Build history of the part. All positions in model axes, mm. Round coordinates to 2 decimals unless told otherwise and drop trailing zeros. Use a Markdown table: item, result. Add a question column.
Item 1: Probe L1, parallel to Z at x = -24.5, y = 2; L2, parallel to X at y = 2.5, z = -13.25; L3, parallel to Z at x = 23.5, y = 1.25. List the from-to ranges inside material, lowest first.
Item 2: Two-plate mould, pull along X, no slides. Class faces 1 (the face through (127, 5, 1)), 2 (the face through (-127, 5, 1)), 3 (the face through (-99.543, 4.829, -1.041)): released by +X, released by -X, zero draft, split by the parting line, or undercut.
Item 3: Slice it at A-A, the plane y = 3.75. State how many separate pieces and enclosed holes the cut face has, plus the area to 3 significant figures.
from build123d import *

# Parameters (mm, degrees)
SKETCH1_W                      = 254
SKETCH1_H                      = 114.3
BOSS_EXTRUDE1_DEPTH            = 9.525
F_3_8_CLEARANCE_HOLE1_D        = 9.8044
F_3_8_CLEARANCE_HOLE1_DEPTH    = 10
F_3_8_CLEARANCE_HOLE1_TIP      = 2.945538927
M2_5_CLEARANCE_HOLE3_D         = 3.1
M2_5_CLEARANCE_HOLE3_DEPTH     = 10
M2_5_CLEARANCE_HOLE3_TIP       = 0.931333959
FILLET1_R                      = 2
M3_CLEARANCE_HOLE4_D           = 3.4
M3_CLEARANCE_HOLE4_DEPTH       = 10
M3_CLEARANCE_HOLE4_TIP         = 1.021463052
SKETCH22_R                     = 8
CUT_EXTRUDE1_DEPTH             = 140.5917194
M3_CLEARANCE_HOLE5_D           = 3.6
M3_CLEARANCE_HOLE5_DEPTH       = 10
M3_CLEARANCE_HOLE5_TIP         = 1.081549114
M2_5_CLEARANCE_HOLE4_OUTLINE_R = 1.55
M2_5_CLEARANCE_HOLE4_DEPTH     = 9.525


# Read off the part's stored shape, not the designer's step: M2.5 Clearance Hole4
with BuildPart() as part:
    # Sketch1 → Boss-Extrude1 (new body)
    with BuildSketch(Plane(origin=(0, 0, 0), x_dir=(1, 0, 0), z_dir=(0, 1, 0))):
        Rectangle(SKETCH1_W, SKETCH1_H)
    extrude(amount=BOSS_EXTRUDE1_DEPTH)

    # 3/8 Clearance Hole1
    with Locations(Plane(origin=(0, 9.525, 0), x_dir=(1, 0, 0), z_dir=(0, 1, 0))):
        with Locations((112.7125, 42.8625), (112.7125, -42.8675), (-112.7175, 42.8625), (-112.7175, -42.8675)):
            Hole(F_3_8_CLEARANCE_HOLE1_D / 2, depth=F_3_8_CLEARANCE_HOLE1_DEPTH)
            with Locations((0, 0, -(F_3_8_CLEARANCE_HOLE1_DEPTH + F_3_8_CLEARANCE_HOLE1_TIP / 2))):  # 118° drill point
                Cone(0, F_3_8_CLEARANCE_HOLE1_D / 2, F_3_8_CLEARANCE_HOLE1_TIP, mode=Mode.SUBTRACT)

    # M2.5 Clearance Hole3
    with Locations(Plane(origin=(0, 9.525, 0), x_dir=(1, 0, 0), z_dir=(0, 1, 0))):
        with Locations((24.5, 19), (-24.5, -39), (24.5, -39), (-24.5, 19)):
            Hole(M2_5_CLEARANCE_HOLE3_D / 2, depth=M2_5_CLEARANCE_HOLE3_DEPTH)
            with Locations((0, 0, -(M2_5_CLEARANCE_HOLE3_DEPTH + M2_5_CLEARANCE_HOLE3_TIP / 2))):  # 118° drill point
                Cone(0, M2_5_CLEARANCE_HOLE3_D / 2, M2_5_CLEARANCE_HOLE3_TIP, mode=Mode.SUBTRACT)

    # Fillet1
    fillet1_edges = [part.edges().sort_by_distance(p)[0] for p in [
        (127, 4.7625, 57.15),
        (-127, 4.7625, 57.15),
        (-127, 4.7625, -57.15),
        (127, 4.7625, -57.15),
    ]]
    fillet(fillet1_edges, radius=FILLET1_R)

    # M3 Clearance Hole4
    with Locations(Plane(origin=(0, 9.525, 0), x_dir=(1, 0, 0), z_dir=(0, 1, 0))):
        with Locations((-90.2, -20.8), (-88.35, 29.15), (-58.8, 13.25), (-46, -20.8)):
            Hole(M3_CLEARANCE_HOLE4_D / 2, depth=M3_CLEARANCE_HOLE4_DEPTH)
            with Locations((0, 0, -(M3_CLEARANCE_HOLE4_DEPTH + M3_CLEARANCE_HOLE4_TIP / 2))):  # 118° drill point
                Cone(0, M3_CLEARANCE_HOLE4_D / 2, M3_CLEARANCE_HOLE4_TIP, mode=Mode.SUBTRACT)

    # Sketch22 → Cut-Extrude1 (cut, through all)
    with BuildSketch(Plane(origin=(0, 9.525, 0), x_dir=(1, 0, 0), z_dir=(0, 1, 0))):
        with Locations(Location((-107.475, 0, 0), (0, 0, 270))):
            Circle(SKETCH22_R)
    extrude(amount=-CUT_EXTRUDE1_DEPTH, mode=Mode.SUBTRACT)

    # M3 Clearance Hole5
    with Locations(Plane(origin=(0, 9.525, 0), x_dir=(1, 0, 0), z_dir=(0, 1, 0))):
        with Locations((61.84, 40.64), (61.84, -40.64), (82.16, -40.64), (82.16, 40.64)):
            Hole(M3_CLEARANCE_HOLE5_D / 2, depth=M3_CLEARANCE_HOLE5_DEPTH)
            with Locations((0, 0, -(M3_CLEARANCE_HOLE5_DEPTH + M3_CLEARANCE_HOLE5_TIP / 2))):  # 118° drill point
                Cone(0, M3_CLEARANCE_HOLE5_D / 2, M3_CLEARANCE_HOLE5_TIP, mode=Mode.SUBTRACT)

    # M2.5 Clearance Hole4 outline → M2.5 Clearance Hole4 (cut)
    with BuildSketch(Plane(origin=(0, 0, 0), x_dir=(1, 0, 0), z_dir=(0, 1, 0))):
        with Locations((-10.16, 6.35)):
            Circle(M2_5_CLEARANCE_HOLE4_OUTLINE_R)
        with Locations((10.16, 6.35)):
            Circle(M2_5_CLEARANCE_HOLE4_OUTLINE_R)
        with Locations((10.16, -6.35)):
            Circle(M2_5_CLEARANCE_HOLE4_OUTLINE_R)
        with Locations((-10.16, -6.35)):
            Circle(M2_5_CLEARANCE_HOLE4_OUTLINE_R)
    extrude(amount=M2_5_CLEARANCE_HOLE4_DEPTH, mode=Mode.SUBTRACT)


solid = part.part
Check sheet entries:
| question | item | result |
|---|---|---|
| 1 | L1 | -57.15 to -20.55, -17.45 to 37.45, 40.55 to 57.15 |
| 1 | L2 | -127 to -60.5, -57.1 to 127 |
| 1 | L3 | -57.15 to -20.18, -17.82 to 37.82, 40.18 to 57.15 |
| 2 | face 1 | released by +X |
| 2 | face 2 | released by -X |
| 2 | face 3 | undercut |
| 3 | separate pieces | 1 |
| 3 | enclosed holes | 21 |
| 3 | area | 28,400 mm2 |
